Autodesk Inventor part; units mm, degrees
ref_plane "YZ Plane" through (0, 0, 0) normal (1, 0, 0) x (0, 1, 0)
ref_plane "XZ Plane" through (0, 0, 0) normal (0, 1, 0) x (-1, 0, 0)
ref_plane "XY Plane" through (0, 0, 0) normal (0, 0, 1) x (1, 0, 0)
sketch "Sketch1" plane through (0, 0, 0) normal (0, 0, 1) x (1, 0, 0)
  line L0 (-50.75, 79.75) -> (50.75, 79.75)
  line L1 (54.75, 75.75) -> (54.75, -75.75)
  line L2 (50.75, -79.75) -> (-50.75, -79.75)
  line L3 (-54.75, -75.75) -> (-54.75, 75.75)
  arc A0 (-50.75, 79.75) -> (-54.75, 75.75) centre (-50.75, 75.75) ccw
  arc A1 (-54.75, -75.75) -> (-50.75, -79.75) centre (-50.75, -75.75) ccw
  arc A2 (50.75, -79.75) -> (54.75, -75.75) centre (50.75, -75.75) ccw
  arc A3 (54.75, 75.75) -> (50.75, 79.75) centre (50.75, 75.75) ccw
  point P0 (0, 0)
  point P1 (-54.75, 79.75)
  point P2 (54.75, 79.75)
  point P3 (-54.75, -79.75)
  dimension "d0" = 109.5
  dimension "d1" = 159.5
  dimension "d2" = 54.75
  dimension "d3" = 79.75
  dimension "d4" = 4
extrude "xyAttach" add sketch "Sketch1" along normal blind 3
sketch "Sketch2" plane through (0, 0, 3) normal (0, 0, 1) x (1, 0, 0)
  line L0 (-50.75, 79.75) -> (50.75, 79.75)
  line L1 (54.75, 75.75) -> (54.75, -75.75)
  line L2 (50.75, -79.75) -> (-50.75, -79.75)
  line L3 (-54.75, -75.75) -> (-54.75, 75.75)
  line L4 (50.75, 79.75) -> (-50.75, 79.75)
  line L5 (-54.75, 75.75) -> (-54.75, -75.75)
  line L6 (-50.75, -79.75) -> (50.75, -79.75)
  line L7 (54.75, -75.75) -> (54.75, 75.75)
  arc A0 (-50.75, 79.75) -> (-54.75, 75.75) centre (-50.75, 75.75) ccw
  arc A1 (-54.75, -75.75) -> (-50.75, -79.75) centre (-50.75, -75.75) ccw
  arc A2 (50.75, -79.75) -> (54.75, -75.75) centre (50.75, -75.75) ccw
  arc A3 (54.75, 75.75) -> (50.75, 79.75) centre (50.75, 75.75) ccw
  line L8 (-48.75, 77.75) -> (48.75, 77.75)
  line L9 (52.75, 73.75) -> (52.75, -73.75)
  line L10 (48.75, -77.75) -> (-48.75, -77.75)
  line L11 (-52.75, -73.75) -> (-52.75, 73.75)
  arc A4 (-48.75, 77.75) -> (-52.75, 73.75) centre (-48.75, 73.75) ccw
  arc A5 (-52.75, -73.75) -> (-48.75, -77.75) centre (-48.75, -73.75) ccw
  arc A6 (48.75, -77.75) -> (52.75, -73.75) centre (48.75, -73.75) ccw
  arc A7 (52.75, 73.75) -> (48.75, 77.75) centre (48.75, 73.75) ccw
  point P0 (0, 0)
  dimension "d7" = 4
  dimension "d8" = 4
  dimension "d9" = 2
  dimension "d10" = 2
  dimension "d11" = 2
  dimension "d12" = 2
extrude "spillExtrusion" add sketch "Sketch2" along normal blind 2
sketch "Sketch3" plane through (0, 0, 3) normal (0, 0, 1) x (1, 0, 0)
  line L0 (-33, 40) -> (33, 40)
  line L1 (35, 38) -> (35, -38)
  line L2 (33, -40) -> (-33, -40)
  line L3 (-35, -38) -> (-35, 38)
  arc A0 (-33, 40) -> (-35, 38) centre (-33, 38) ccw
  arc A1 (-35, -38) -> (-33, -40) centre (-33, -38) ccw
  arc A2 (35, 38) -> (33, 40) centre (33, 38) ccw
  arc A3 (33, -40) -> (35, -38) centre (33, -38) ccw
  point P0 (0, 0)
  point P1 (-35, 40)
  point P2 (35, -40)
  point P3 (35, 40)
  dimension "d15" = 70
  dimension "d16" = 35
  dimension "d17" = 80
  dimension "d18" = 40
  dimension "d19" = 2
extrude "chamberWallExtrusion" add sketch "Sketch3" along normal blind 50
sketch "Sketch4" plane through (0, 0, 53) normal (0, 0, 1) x (1, 0, 0)
  line L0 (-27, 36.5) -> (29.5, 36.5)
  line L1 (31.5, 34.5) -> (31.5, -34.5)
  line L2 (29.5, -36.5) -> (-27, -36.5)
  line L3 (-29, -34.5) -> (-29, 34.5)
  arc A0 (-27, 36.5) -> (-29, 34.5) centre (-27, 34.5) ccw
  arc A1 (-29, -34.5) -> (-27, -36.5) centre (-27, -34.5) ccw
  arc A2 (29.5, -36.5) -> (31.5, -34.5) centre (29.5, -34.5) ccw
  arc A3 (31.5, 34.5) -> (29.5, 36.5) centre (29.5, 34.5) ccw
  line L4 (33, 40) -> (-33, 40)
  line L5 (35, -38) -> (35, 38)
  line L6 (-33, -40) -> (33, -40)
  line L7 (-35, 38) -> (-35, -38)
  point P0 (0, 0)
  dimension "d22" = 2
  dimension "d23" = 3.5
  dimension "d24" = 3.5
  dimension "d25" = 3.5
  dimension "d26" = 6
extrude "chamberInteriorExtrusion" cut sketch "Sketch4" against normal blind 35.5
sketch "Sketch5" plane through (-29, -34.5, 53) normal (1, 0, 0) x (0, 0, -1)
  line L0 (5.5, 3.25) -> (35.5, 3.25)
  line L1 (35.5, 3.25) -> (35.5, 65.75)
  line L2 (35.5, 65.75) -> (5.5, 65.75)
  line L3 (5.5, 65.75) -> (5.5, 3.25)
  line L4 (48, 110.25) -> (48, -41.25)
  point P0 (53, 34.5)
  dimension "d29" = 62.5
  dimension "d30" = 30
  dimension "d31" = 31.25
  dimension "d32" = 42.5
extrude "rectCoverSlipMountExtrusion" cut sketch "Sketch5" against normal blind 2
sketch "Sketch6" plane through (-31, -34.5, 53) normal (1, 0, 0) x (0, 0, -1)
  line L0 (10.5, 7) -> (30.5, 7)
  line L1 (30.5, 7) -> (30.5, 62)
  line L2 (30.5, 62) -> (10.5, 62)
  line L3 (10.5, 62) -> (10.5, 7)
  line L4 (48, -39.25) -> (48, 108.25)
  point P0 (53, 34.5)
  dimension "d35" = 55
  dimension "d36" = 20
  dimension "d37" = 37.5
  dimension "d38" = 27.5
extrude "rectCoverSlipWindow" cut sketch "Sketch6" against normal up to surface (4 mm away)
sketch "Sketch7" plane through (-35, -38, 3) normal (-1, 0, 0) x (0, 0, 1)
  line L0 (50, 73) -> (2, 73)
  line L1 (2, 73) -> (2, 3)
  line L2 (2, 3) -> (50, 3)
  line L3 (50, 3) -> (50, 73)
  line L4 (50, 76) -> (50, 0)
  line L5 (2, 113.75) -> (2, -37.75)
  point P0 (-3, 38)
  dimension "d41" = 70
  dimension "d42" = 35
extrude "illObjExtrusion" cut sketch "Sketch7" against normal blind 2
sketch "Sketch8" plane through (-27, -36.5, 53) normal (0, 1, 0) x (1, 0, 0)
  line L0 (47.5, 33) -> (2.5, 33)
  line L1 (2.5, 33) -> (2.5, 8)
  line L2 (2.5, 8) -> (47.5, 8)
  line L3 (47.5, 8) -> (47.5, 33)
  point P0 (27, 53)
  point P1 (-27.75, 48)
  point P2 (-2, 0)
  dimension "d46" = 45
  dimension "d47" = 25
  dimension "d48" = 40
  dimension "d69" = 4.5
extrude "viewingWindowCoverslipMount" cut sketch "Sketch8" against normal blind 2
sketch "Sketch9" plane through (-27, -38.5, 53) normal (0, 1, 0) x (1, 0, 0)
  line L0 (7.5, 29) -> (42.5, 29)
  line L1 (42.5, 29) -> (42.5, 12)
  line L2 (42.5, 12) -> (7.5, 12)
  line L3 (7.5, 12) -> (7.5, 29)
  line L4 (-23.75, 48) -> (77.75, 48)
  line L5 (2.5, 8) -> (2.5, 33)
  point P0 (27, 53)
  point P1 (-2, 0)
  dimension "d52" = 35
  dimension "d53" = 17
  dimension "d55" = 36
  dimension "d71" = 5
extrude "viewingWindowExt" cut sketch "Sketch9" against normal up to surface (1.5 mm away)
sketch "Sketch10" plane through (0, 0, 17.5) normal (0, 0, 1) x (1, 0, 0)
  circle A0 centre (-15, 0) radius 2.825
  circle A1 centre (0, 15) radius 2.825
  circle A2 centre (15, 0) radius 2.825
  circle A3 centre (0, -15) radius 2.825
  circle A4 centre (0, 0) radius 2.825
  dimension "d58" = 5.65
  dimension "d59" = 5.65
  dimension "d60" = 5.65
  dimension "d61" = 5.65
  dimension "d62" = 5.65
  dimension "d63" = 15
  dimension "d64" = 15
  dimension "d65" = 15
  dimension "d66" = 15
extrude "sampleMountExt" cut sketch "Sketch10" against normal blind 2
equation "\"d10\" = d9"
equation "\"d11\" = d9"
equation "\"d12\" = d9"
equation "\"d24\" = d23"
equation "\"d25\" = d23"
equation "\"d59\" = d58"
equation "\"d60\" = d58"
equation "\"d61\" = d58"
equation "\"d62\" = d58"
properties part number "sampleChamberExt_v1"
Geometry check sheet. Reference: the model listing, model coordinates, mm. A direction names the side the tool comes from. Give positions to 0.01 mm unless a question says otherwise; leave off trailing zeros. Write each loop counter-clockwise with the first axis right and the second up, starting at its lowest first coordinate (ties: lowest second). Pieces come first, ordered by that corner, then holes. Notation, with made-up numbers: (-26, 24) -> (29, 24) arc R14 ccw to (29, 42) -> close; hole circle Ø4 at (-8, 11.5). An arc over 180 degrees is marked (long way). One line per question, with ' | ' between items.
Item 1: Depth check by flat-ended pin: pin 1 (4 mm diameter, centred on x = -23, z = 11.5, fed in from -Y); pin 2 (10 mm diameter, centred on y = 0, z = 40, fed in from +X); pin 3 (5 mm diameter, centred on x = -15, z = 12, fed in from +Y); pin 4 (12 mm diameter, centred on y = -56, z = 12, fed in from -X). Enter the tip coordinate at first touch or a pass-through.
Determined:
pin 1: y = -40 | pin 2: x = 35 | pin 3: y = 40 | pin 4: through
Item 2: Sectioned sample at D-D, the plane y = 61. Record the boundary of the cut face in (x, z), plus the area to 4 significant figures.
Determined:
outline: (-54.75, 0) -> (54.75, 0) -> (54.75, 5) -> (52.75, 5) -> (52.75, 3) -> (-52.75, 3) -> (-52.75, 5) -> (-54.75, 5) -> close | area: 336.5 mm^2
Item 3: Access from +Z, -Z, +X, -X, +Y, -Y to the whole of each face (thin tool, end or side, straight path). Record for faces 4 (the flat face through (-2, -38.5, 21)), 5 (the flat face through (-33, 0, 18)), 6 (the flat face through (15, 0, 15.5)).
Determined:
face 4: none | face 5: +Z, -X | face 6: +Z
Item 4: Sectioned sample at B-B, the plane x = 42.5. Record the boundary of the cut face in (y, z), plus the area to 4 significant figures.
Determined:
outline: (-79.75, 0) -> (79.75, 0) -> (79.75, 5) -> (77.75, 5) -> (77.75, 3) -> (-77.75, 3) -> (-77.75, 5) -> (-79.75, 5) -> close | area: 486.5 mm^2
Item 5: Draft check along Y on faces 1 (the flat face through (-1, 79.75, 2)), 2 (the cylindrical face through (53.609, -78.547, 2.465)), 3 (the cylindrical face through (51.547, 76.609, 3.986)). Enter one of: released by +Y, released by -Y, zero draft, split by the parting line, or undercut.
Determined:
face 1: released by +Y | face 2: released by -Y | face 3: undercut
Item 6: Sectioned sample at C-C, the plane z = 9. Record the boundary of the cut face in (x, y).
Determined:
outline: (-35, -38) arc R2 ccw to (-33, -40) -> (33, -40) arc R2 ccw to (35, -38) -> (35, 38) arc R2 ccw to (33, 40) -> (-33, 40) arc R2 ccw to (-35, 38) -> (-35, 35) -> (-33, 35) -> (-33, -35) -> (-35, -35) -> close
Item 7: Scan lines: line 1 along Y through (x, z) = (0, 17) (3 decimals); line 2 along Y through (x, z) = (15, 16) (3 decimals); line 3 along X through (y, z) = (34, 48). Record each from-to range of solid material in increasing order.
Determined:
line 1: -40 to -17.825, -12.175 to -2.825, 2.825 to 12.175, 17.825 to 40 | line 2: -40 to -2.825, 2.825 to 40 | line 3: -33 to -29, 31.5 to 35
Item 8: Sectioned sample at A-A, the plane y = -15. Record the boundary of the cut face in (x, z) (3 decimals), plus the area to 3 significant figures.
Determined:
outline: (-54.75, 0) -> (54.75, 0) -> (54.75, 5) -> (52.75, 5) -> (52.75, 3) -> (35, 3) -> (35, 53) -> (31.5, 53) -> (31.5, 17.5) -> (2.825, 17.5) -> (2.825, 15.5) -> (-2.825, 15.5) -> (-2.825, 17.5) -> (-31, 17.5) -> (-31, 22.5) -> (-33, 22.5) -> (-33, 5) -> (-35, 5) -> (-35, 3) -> (-52.75, 3) -> (-52.75, 5) -> (-54.75, 5) -> close; (-33, 42.5) -> (-31, 42.5) -> (-31, 47.5) -> (-29, 47.5) -> (-29, 53) -> (-33, 53) -> close | area: 1,480 mm^2
